Check sheet for the modelled part. Datum: model origin and axes. Units: mm. Face numbers are marked on the shaded views. A direction names the side the tool comes from. Give positions to 0.01 mm unless a question says otherwise; leave off trailing zeros. Loops run counter-clockwise (first coordinate to the right, second up) from the corner with the lowest first, then second, coordinate; pieces in that order, holes last. Notation, with made-up numbers: M 1,64.5 L 36,64.5 A20 ccw 36,103.5 Z; hole C 16,6.25 d2. An arc over 180 degrees is marked long. Write each question's results on one line, items separated by ' | '. Start each with the question number.
1. Sectioned sample at B-B on y = -30. Record the cut outline in (x, z) (3 decimals), and give its area (3 significant figures).
2. Sectioned sample at D-D on y = 59.5. Record the cut outline in (x, z) (3 decimals).
3. Draft check along Y on the marked faces 3 and 4. Enter one of: pulls with the +Y half, pulls with the -Y half, needs draft (parallel to the pull), parting line crosses it, or undercut.
4. Material ranges on line 1 along X through (y, z) = (3, 6.25) (1 decimal); line 2 along Y through (x, z) = (-9, 10); line 3 along X through (y, z) = (-36, 5.75) (3 decimals), recorded low to high.
5. Tool access check on the marked faces 1 and 2. Record the directions out of +Z, -Z, +X, -X, +Y, -Y that give a thin tool (end or side, any length) a straight path to the whole face; none if there is none.
6. Sectioned sample at C-C on x = -16. Record the cut outline in (y, z).
7. Go/stop test with a flat-tipped pin: pin 1 (12 mm diameter, centred on x = -26, y = -12.5, fed in from -Z). Record where the tip stops, or that it passes through.
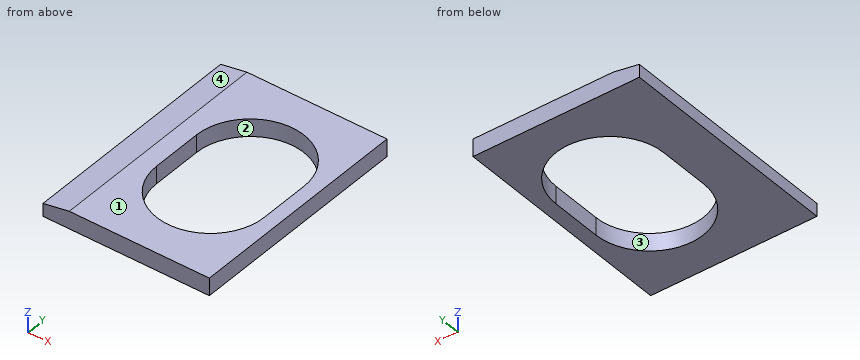
```python
from build123d import *

# Parameters (mm, degrees)
SKETCH1_W           = 120.65
SKETCH1_H           = 165.1
BOSS_EXTRUDE1_DEPTH = 12.7
CUT_EXTRUDE1_REACH  = 105.029
CUT_EXTRUDE2_REACH  = 178.234


with BuildPart() as part:
    # Sketch1 → Boss-Extrude1 (new body)
    with BuildSketch(Plane.XY):
        Rectangle(SKETCH1_W, SKETCH1_H)
    extrude(amount=BOSS_EXTRUDE1_DEPTH)

    # Sketch2 → Cut-Extrude1 (cut, up to next)
    with BuildSketch(Plane.XY.offset(12.7), mode=Mode.PRIVATE) as cut_extrude1_sk1:
        with BuildLine():
            Line((50.1015, 18.5039), (50.1015, -18.5039))
            ThreePointArc((50.1015, -18.5039), (11.0998, -57.5056), (-27.9019, -18.5039))
            Line((-27.9019, -18.5039), (-27.9019, 18.5039))
            ThreePointArc((-27.9019, 18.5039), (11.0998, 57.5056), (50.1015, 18.5039))
        make_face()
    cut_extrude1_tool1 = extrude(cut_extrude1_sk1.sketch, amount=-CUT_EXTRUDE1_REACH, mode=Mode.PRIVATE) & part.part
    add(cut_extrude1_tool1.solids().sort_by_distance((11.0998, 0, 12.7))[0], mode=Mode.SUBTRACT)

    # Sketch3 → Cut-Extrude2 (cut, up to next)
    with BuildSketch(Plane(origin=(0, 82.55, 0), x_dir=(1, 0, 0), z_dir=(0, 1, 0)), mode=Mode.PRIVATE) as cut_extrude2_sk1:
        Polygon((-41.276197421, -12.7), (-60.325, -9.341182155), (-60.325, -12.7), align=None)
    cut_extrude2_tool1 = extrude(cut_extrude2_sk1.sketch, amount=-CUT_EXTRUDE2_REACH, mode=Mode.PRIVATE) & part.part
    add(cut_extrude2_tool1.solids().sort_by_distance((-53.975399, 82.55, 11.580394))[0], mode=Mode.SUBTRACT)


solid = part.part
```
Output values:
1) outline: M -60.325,0 L -26.169,0 L -26.169,12.7 L -41.276,12.7 L -60.325,9.341 Z; M 48.369,0 L 60.325,0 L 60.325,12.7 L 48.369,12.7 Z | area: 554 mm2
2) outline: M -60.325,0 L 60.325,0 L 60.325,12.7 L -41.276,12.7 L -60.325,9.341 Z
3) face 3: undercut | face 4: needs draft
4) line 1: -60.3 to -27.9, 50.1 to 60.3 | line 2: -82.55 to -51.93, 51.93 to 82.55 | line 3: -60.325 to -23.757, 45.957 to 60.325
5) face 1: +Z, +X, -X, +Y, -Y | face 2: +Z, -Z
6) outline: M -82.55,0 L -46.55,0 L -46.55,12.7 L -82.55,12.7 Z; M 46.55,0 L 82.55,0 L 82.55,12.7 L 46.55,12.7 Z
7) pin 1: z = 0
